For this review, take the finished solid that the model builds, in its own axes (mm). A direction names the side the tool comes from. Give positions to 0.01 mm unless a question says otherwise; leave off trailing zeros. Loops run counter-clockwise (first coordinate to the right, second up) from the corner with the lowest first, then second, coordinate; pieces in that order, holes last. Notation, with made-up numbers: (44.25, 88) - (71.25, 88) arc R33 ccw to (71.25, 124) - close; hole circle Ø7 at (-25.75, 26.25). An arc over 180 degrees is marked (long way). Answer in a Markdown table with one row per item.
```python
from build123d import *

# Parameters (mm, degrees)
BOSS_EXTRUDE3_DEPTH = 3.175
SKETCH3_W           = 12.7
SKETCH3_H           = 3.175
BOSS_EXTRUDE4_DEPTH = 47.625
SKETCH4_R           = 3.175
CUT_EXTRUDE1_DEPTH  = 16.256


with BuildPart() as part:
    # Sketch1 → Boss-Extrude3 (new body)
    with BuildSketch(Plane(origin=(0, 0, 0), x_dir=(0, 0, -1), z_dir=(1, 0, 0))):
        with BuildLine():
            ThreePointArc((-15.875, -3.175), (-18.12006403, 2.24506403), (-12.7, 0))
            Line((-12.7, 0), (0, 0))
            Line((0, 0), (0, 12.7))
            Line((0, 12.7), (-22.115038819, 12.7))
            Line((-22.115038819, 12.7), (-27.887655145, 12.7))
            Line((-27.887655145, 12.7), (-27.887655145, -12.7))
            Line((-27.887655145, -12.7), (-15.875, -12.7))
            Line((-15.875, -12.7), (-15.875, -3.175))
        make_face()
        with BuildLine():
            Line((0, 12.7), (0, 0))
            Line((0, 0), (12.7, 0))
            ThreePointArc((12.7, 0), (13.62993597, 2.24506403), (15.875, 3.175))
            Line((15.875, 3.175), (15.875, 12.7))
            Line((15.875, 12.7), (0, 12.7))
        make_face()
        with BuildLine():
            Line((0, 0), (-12.7, 0))
            ThreePointArc((-12.7, 0), (-13.62993597, -2.24506403), (-15.875, -3.175))
            Line((-15.875, -3.175), (-15.875, -12.7))
            Line((-15.875, -12.7), (22.115038819, -12.7))
            Line((22.115038819, -12.7), (27.887655145, -12.7))
            Line((27.887655145, -12.7), (27.887655145, 12.7))
            Line((27.887655145, 12.7), (15.875, 12.7))
            Line((15.875, 12.7), (15.875, 3.175))
            ThreePointArc((15.875, 3.175), (18.12006403, 2.24506403), (19.05, 0))
            ThreePointArc((19.05, 0), (15.875, -3.175), (12.7, 0))
            Line((12.7, 0), (0, 0))
        make_face()
    extrude(amount=BOSS_EXTRUDE3_DEPTH)

    # Sketch3 → Boss-Extrude4 (add)
    with BuildSketch(Plane(origin=(3.175, 0, 0), x_dir=(0, 0, -1), z_dir=(1, 0, 0))):
        with Locations((-6.35, -11.1125)):
            Rectangle(SKETCH3_W, SKETCH3_H)
        with Locations((6.35, -11.1125)):
            Rectangle(SKETCH3_W, SKETCH3_H)
    extrude(amount=BOSS_EXTRUDE4_DEPTH)

    # Sketch4 → Cut-Extrude1 (cut)
    with BuildSketch(Plane(origin=(0, -9.525, 0), x_dir=(1, 0, 0), z_dir=(0, 1, 0))):
        with Locations(Location((19.05, 0, 0), (0, 0, 270))):
            Circle(SKETCH4_R)
        with Locations(Location((34.925, 0, 0), (0, 0, 270))):
            Circle(SKETCH4_R)
    extrude(amount=-CUT_EXTRUDE1_DEPTH, mode=Mode.SUBTRACT)


solid = part.part
```
1. We need section C-C, the plane z = -7.5. Give the boundary of the cut face in (x, y) (3 decimals).
Values:
| item | result |
|---|---|
| outline | (0, -12.7) - (50.8, -12.7) - (50.8, -9.525) - (3.175, -9.525) - (3.175, 12.7) - (0, 12.7) - close |
2. We need section B-B, the plane z = 0. Give the boundary of the cut face in (x, y) (3 decimals), and give its area (3 significant figures).
Values:
| item | result |
|---|---|
| outline | (0, -12.7) - (15.875, -12.7) - (15.875, -9.525) - (3.175, -9.525) - (3.175, 12.7) - (0, 12.7) - close; (22.225, -12.7) - (31.75, -12.7) - (31.75, -9.525) - (22.225, -9.525) - close; (38.1, -12.7) - (50.8, -12.7) - (50.8, -9.525) - (38.1, -9.525) - close |
| area | 192 mm^2 |
3. Mouldability with a two-part tool opening along Z and no side actions: class faces 4 (the face through (3.175, 0, 0)), 5 (the face through (15.95, -11.09, -0.69)), 6 (the face through (27, -11, 12.7)) as released by +Z, released by -Z, zero draft, split by the parting line, or undercut.
Values:
| item | result |
|---|---|
| face 4 | zero draft |
| face 5 | undercut |
| face 6 | released by +Z |
4. Wall thickness on line 1 (X direction, y = -10.4, z = 0) (3 decimals); line 2 (Z direction, x = 29, y = -11); line 3 (X direction, y = -3.5, z = -23) (3 decimals): over which ranges is each line inside the solid? List them lowest first. Write a range as [from, to].
Values:
| item | result |
|---|---|
| line 1 | x = [0, 15.875], [22.225, 31.75], [38.1, 50.8] |
| line 2 | z = [-12.7, 12.7] |
| line 3 | x = [0, 3.175] |
5. For faces 1 (the face through (2, 12.7, 0)), 2 (the face through (27, -9.525, 0)), 3 (the face through (27, -11, -12.7)), list the 3-axis set-ups (+Z, -Z, +X, -X, +Y, -Y) from which the entire face can be reached by the end or side of a thin tool; tool diameter is ignored.
Values:
| item | result |
|---|---|
| face 1 | +Z, -Z, +X, -X, +Y |
| face 2 | +Z, -Z, +X, +Y |
| face 3 | -Z, +X, +Y, -Y |
6. We need section D-D, the plane x = 34. Give the boundary of the cut face in (y, z) (3 decimals), and give its area (3 significant figures).
Values:
| item | result |
|---|---|
| outline | (-12.7, -12.7) - (-9.525, -12.7) - (-9.525, -3.037) - (-12.7, -3.037) - close; (-12.7, 3.037) - (-9.525, 3.037) - (-9.525, 12.7) - (-12.7, 12.7) - close |
| area | 61.4 mm^2 |
7. We need section A-A, the plane x = 19.05. Give the boundary of the cut face in (y, z) (3 decimals), and give its area (3 significant figures).
Values:
| item | result |
|---|---|
| outline | (-12.7, -12.7) - (-9.525, -12.7) - (-9.525, -3.175) - (-12.7, -3.175) - close; (-12.7, 3.175) - (-9.525, 3.175) - (-9.525, 12.7) - (-12.7, 12.7) - close |
| area | 60.5 mm^2 |
8. Clearance check with flat-ended pins moving along their axes: pin 1 (1.5 mm diameter, centred on x = 26, z = 4, fed in from +Y) (3 decimals); pin 2 (1.5 mm diameter, centred on y = 1, z = 15, fed in from -X); pin 3 (1 mm diameter, centred on x = 24, y = -10.5, fed in from +Z); pin 4 (5 mm diameter, centred on y = 2.5, z = 19.5, fed in from +X) (3 decimals). State where each tip first meets the part, or that it passes through.
Values:
| item | result |
|---|---|
| pin 1 | stops at y = -9.525 |
| pin 2 | passes through |
| pin 3 | stops at z = 12.7 |
| pin 4 | stops at x = 3.175 |
